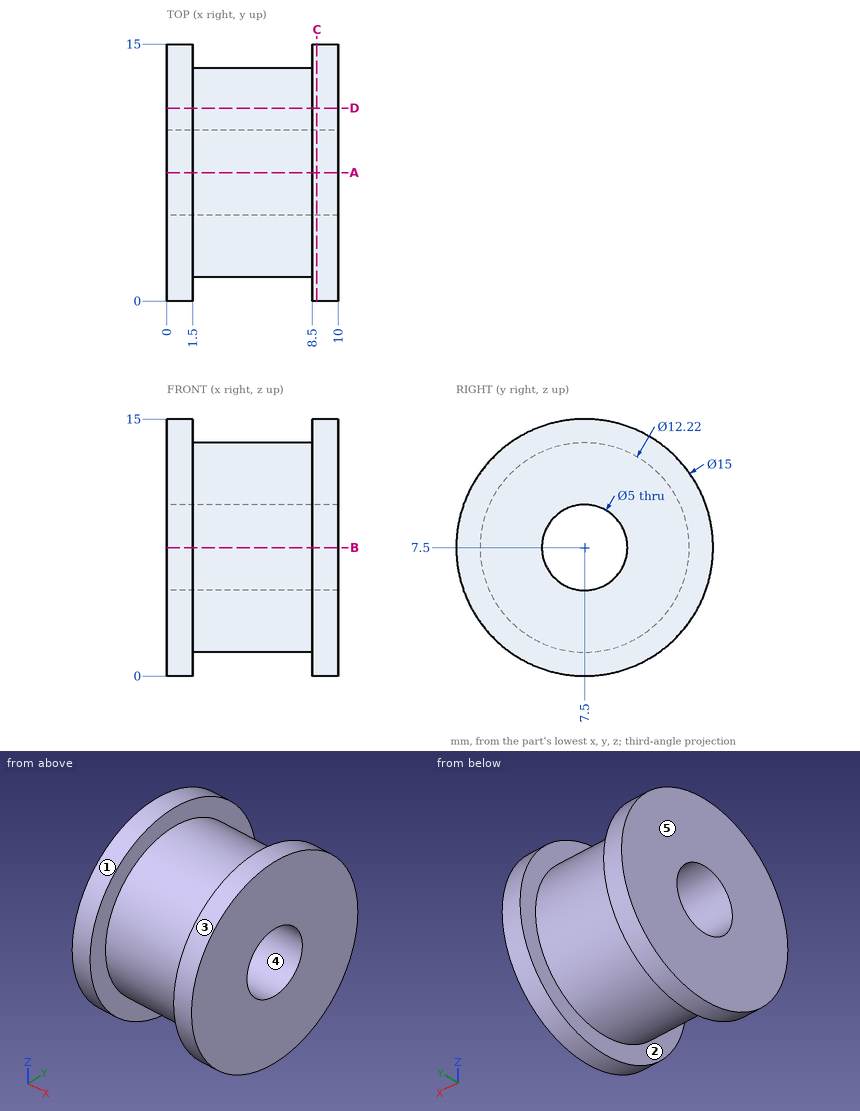
Verification items for this drawing (mm, ordinates from the low corner). A direction names the side the tool comes from. Give positions to 0.01 mm unless a question says otherwise; leave off trailing zeros. Write each loop counter-clockwise with the first axis right and the second up, starting at its lowest first coordinate (ties: lowest second). Pieces come first, ordered by that corner, then holes.
1) Go/stop test with flat-tipped pins: pin 1 Ø4 at (y, z) = (7.5, 7.5) entering from +X; pin 2 Ø2 at (x, y) = (6.5, 2.5) entering from +Z; pin 3 Ø5 at (x, z) = (3, 5) entering from -Y; pin 4 Ø4 at (x, z) = (3, 4) entering from -Y. Record where each tip stops, or that it passes through.
Values follow:
pin 1: passes through
pin 2: stops at z = 12.12
pin 3: stops at y = 0.02
pin 4: stops at y = 0.32
2) Thickness scan on line 1 (Z direction, x = 3.25, y = 7.5); line 2 (X direction, y = 9.75, z = 1.5); line 3 (Y direction, x = 7, z = 8.5). Record the ranges inside material, lowest first.
Values follow:
line 1: z = 1.39 to 5, 10 to 13.61
line 2: x = 0 to 1.5, 8.5 to 10
line 3: y = 1.47 to 5.21, 9.79 to 13.53
3) Cross-section at C-C (x = 8.75). Record the boundary of the cut face in (y, z).
Values follow:
outline: circle Ø15 at (7.5, 7.5); hole circle Ø5 at (7.5, 7.5)
4) Cross-section at D-D (y = 11.25). Record the boundary of the cut face in (x, z).
Values follow:
outline: (0, 1) - (1.5, 1) - (1.5, 2.68) - (8.5, 2.68) - (8.5, 1) - (10, 1) - (10, 14) - (8.5, 14) - (8.5, 12.32) - (1.5, 12.32) - (1.5, 14) - (0, 14) - close
5) Set-up check for the marked faces 1 and 2: record each of +Z, -Z, +X, -X, +Y, -Y from which the full face is reachable in a straight line by a thin tool's end or side.
Values follow:
face 1: +X, -X
face 2: none
6) Release check for a two-part mould opening along Z. For the marked faces 3, 4 and 5 record: released by +Z, released by -Z, zero draft, split by the parting line, or undercut.
Values follow:
face 3: split by the parting line
face 4: undercut
face 5: zero draft
7) Cross-section at A-A (y = 7.5). Record the boundary of the cut face in (x, z).
Values follow:
outline: (0, 0) - (1.5, 0) - (1.5, 1.39) - (8.5, 1.39) - (8.5, 0) - (10, 0) - (10, 5) - (0, 5) - close; (0, 10) - (10, 10) - (10, 15) - (8.5, 15) - (8.5, 13.61) - (1.5, 13.61) - (1.5, 15) - (0, 15) - close
